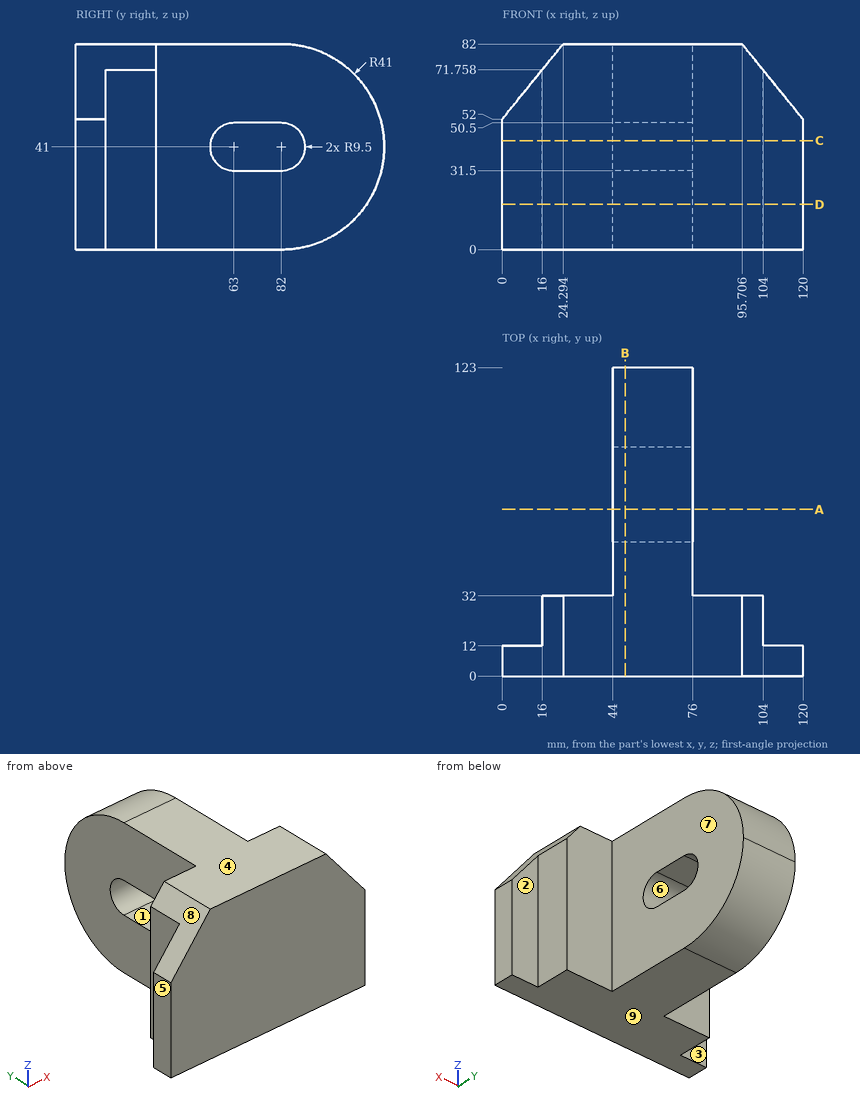
Can you work these out from the drawing? Everything is in mm from the part's minimum corner. A direction names the side the tool comes from. Round coordinates to 2 decimals unless told otherwise and drop trailing zeros. Write each loop counter-clockwise with the first axis right and the second up, starting at its lowest first coordinate (ties: lowest second). Pieces come first, ordered by that corner, then holes. Notation, with made-up numbers: (55, -26) - (113, -26) arc R14 cw to (113, 0) - close; hole circle Ø10 at (74.5, 10.25). An arc over 180 degrees is marked (long way). Put each result on its own line as item: value. Start each with the question number.
(1) For the marked faces 1, 2, 3, 4 and 5, which set-ups out of +Z, -Z, +X, -X, +Y, -Y let a thin tool reach every point of the face, with its end or its side?
(2) I want a section at C-C, the plane z = 43.5. Please give me the cut outline in (x, y) (1 decimal).
(3) Thinking about a two-plate mould opening in Z: for the marked faces 6, 7, 8 and 9, which applies, released by +Z, released by -Z, zero draft, split by the parting line, or undercut?
(4) I want a section at A-A, the plane y = 66.5. Please give me the cut outline in (x, z), plus the area to 3 significant figures.
(5) I need wall thicknesses on probe 1 along X at (y, z) = (100.5, 73.5); probe 2 along Y at (x, z) = (17.5, 64); probe 3 along Y at (x, z) = (71, 33) (1 decimal). Which ranges of each line are inside material? Lowest first, please.
(6) I want a section at B-B, the plane x = 49. Please give me the cut outline in (y, z).
(7) I want a section at D-D, the plane z = 18. Please give me the cut outline in (x, y).
(8) Will these pins go through, and if not, where does the flat tip stop? pin 1 (4 mm diameter, centred on y = 28.5, z = 26.5, fed in from +X); pin 2 (1 mm diameter, centred on x = 42, y = 56.5, fed in from -Z) (1 decimal); pin 3 (8 mm diameter, centred on x = 103.5, z = 17, fed in from +Y); pin 4 (21 mm diameter, centred on x = 59.5, y = 75.5, fed in from -Z).
Here are the results:
1. face 1: +X, -X
1. face 2: +Z, -Z, +X, +Y
1. face 3: +Z, -Z, -X, +Y
1. face 4: +Z, +X, -X, +Y, -Y
1. face 5: +Z, -Z, -X, +Y, -Y
2. outline: (0, 0) - (120, 0) - (120, 12) - (104, 12) - (104, 32) - (76, 32) - (76, 53.8) - (44, 53.8) - (44, 32) - (16, 32) - (16, 12) - (0, 12) - close; (44, 91.2) - (76, 91.2) - (76, 122.9) - (44, 122.9) - close
3. face 6: undercut
3. face 7: zero draft
3. face 8: released by +Z
3. face 9: released by -Z
4. outline: (44, 0) - (76, 0) - (76, 31.5) - (44, 31.5) - close; (44, 50.5) - (76, 50.5) - (76, 82) - (44, 82) - close
4. area: 2,020 mm^2
5. probe 1: x = 44 to 76
5. probe 2: y = 0 to 32
5. probe 3: y = 0 to 57.9, 87.1 to 122.2
6. outline: (0, 0) - (82, 0) arc R41 ccw to (82, 82) - (0, 82) - close; hole (63, 31.5) - (82, 31.5) arc R9.5 ccw to (82, 50.5) - (63, 50.5) arc R9.5 ccw to start
7. outline: (0, 0) - (120, 0) - (120, 12) - (104, 12) - (104, 32) - (76, 32) - (76, 115.94) - (44, 115.94) - (44, 32) - (16, 32) - (16, 12) - (0, 12) - close
8. pin 1: stops at x = 104
8. pin 2: passes through
8. pin 3: stops at y = 32
8. pin 4: stops at z = 0
